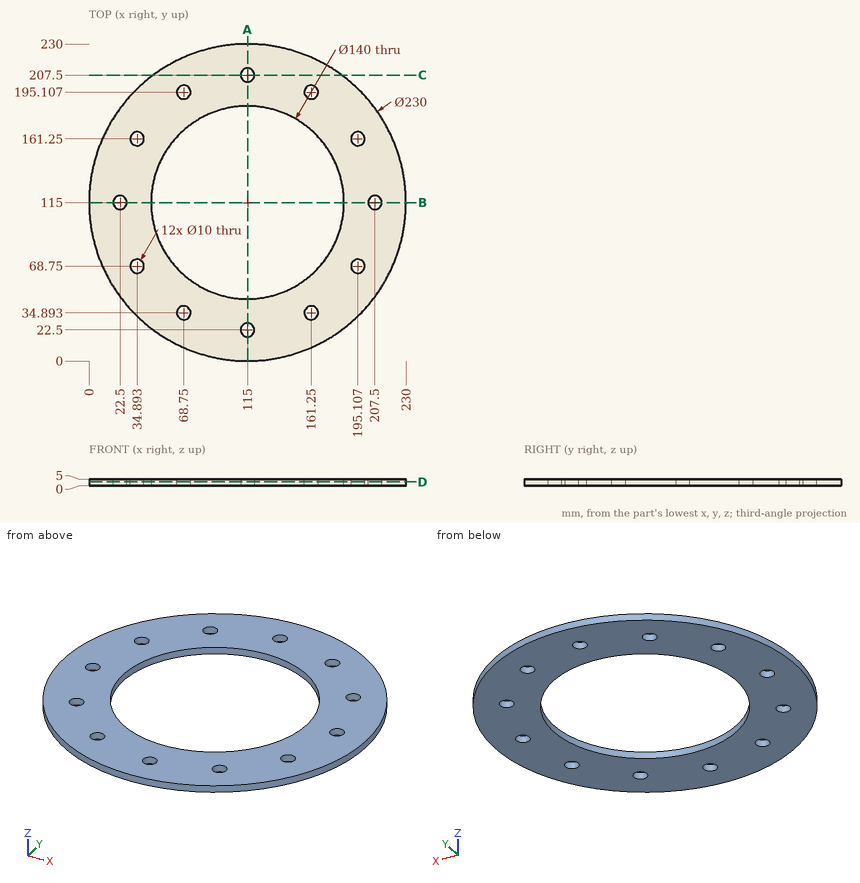
Check sheet for the drawn part. Datum: minimum x, y, z corner. Units: mm. Round coordinates to 2 decimals unless told otherwise and drop trailing zeros. Order: outer loops, then holes, each group sorted by start corner. A loop starts at its lowest first (then second) coordinate and runs counter-clockwise, first axis right, second up. Notation, with made-up numbers: (-26, 58.25) -> (31, 58.25) arc R22 cw to (31, 79.25) -> close; hole circle Ø1 at (55.5, -33). An arc over 180 degrees is marked (long way). Put each result on its own line as item: value.
1) Section check A-A (x = 115). Record the cut outline in (y, z).
Final values:
outline: (0, 0) -> (17.5, 0) -> (17.5, 5) -> (0, 5) -> close; (27.5, 0) -> (45, 0) -> (45, 5) -> (27.5, 5) -> close; (185, 0) -> (202.5, 0) -> (202.5, 5) -> (185, 5) -> close; (212.5, 0) -> (230, 0) -> (230, 5) -> (212.5, 5) -> close
2) Section check D-D (z = 3). Give the number of separate pieces and of enclosed holes in the cut face, then the cut area to 3 significant figures.
Final values:
separate pieces: 1
enclosed holes: 13
area: 25,200 mm^2
3) Material ranges on line 1 (X direction, y = 73, z = 3.6) (1 decimal); line 2 (X direction, y = 194.5, z = 0.55) (1 decimal); line 3 (Y direction, x = 171, z = 1.8) (1 decimal), recorded low to high.
Final values:
line 1: x = 7.9 to 32.3, 37.5 to 59, 171 to 192.5, 197.7 to 222.1
line 2: x = 31.9 to 63.8, 73.7 to 156.3, 166.2 to 198.1
line 3: y = 14.6 to 73, 157 to 215.4
4) Depth check by flat-ended pin: pin 1 (2 mm diameter, centred on x = 126, z = 4.5, fed in from +Y); pin 2 (9 mm diameter, centred on x = 195.11, y = 161.25, fed in from +Z); pin 3 (1.5 mm diameter, centred on y = 102.5, z = 4.5, fed in from -X); pin 4 (1 mm diameter, centred on y = 135.5, z = 3.5, fed in from -X). Enter the tip coordinate at first touch or a pass-through.
Final values:
pin 1: stops at y = 229.56
pin 2: passes through
pin 3: stops at x = 0.6
pin 4: stops at x = 1.75
5) Section check C-C (y = 207.5). Record the cut outline in (x, z), then the cut area to 3 significant figures.
Final values:
outline: (46.67, 0) -> (110, 0) -> (110, 5) -> (46.67, 5) -> close; (120, 0) -> (183.33, 0) -> (183.33, 5) -> (120, 5) -> close
area: 633 mm^2
